from build123d import *

# Parameters (mm, degrees)
SKETCH1_W           = 100
SKETCH1_H           = 1100
BOSS_EXTRUDE1_DEPTH = 200
SKETCH3_W           = 50
SKETCH3_H           = 50
BOSS_EXTRUDE2_DEPTH = 250
FILLET1_R           = 40
BOSS_EXTRUDE3_START = -6
SKETCH4_R           = 20
SKETCH4_R_2         = 15.875
BOSS_EXTRUDE3_DEPTH = 36
CUT_EXTRUDE1_DEPTH  = 20
SKETCH6_W           = 100
SKETCH6_H           = 200
CUT_EXTRUDE2_DEPTH  = 150
SKETCH7_R           = 26
CUT_EXTRUDE3_DEPTH  = 40
SKETCH9_R           = 8
CUT_EXTRUDE5_DEPTH  = 40
SKETCH9_4_R         = 8
CUT_EXTRUDE6_DEPTH  = 40


with BuildPart() as part:
    # Sketch1 → Boss-Extrude1 (new body)
    with BuildSketch(Plane.XY):
        with Locations((-162.86470473, 483.969884115)):
            Rectangle(SKETCH1_W, SKETCH1_H)
    extrude(amount=BOSS_EXTRUDE1_DEPTH)

    # Sketch3 → Boss-Extrude2 (add)
    with BuildSketch(Plane(origin=(-112.86470473, 0, 0), x_dir=(0, 0, -1), z_dir=(1, 0, 0))):
        with Locations((-100, 710.969884115)):
            Rectangle(SKETCH3_W, SKETCH3_H)
    extrude(amount=BOSS_EXTRUDE2_DEPTH)

    # Fillet1
    fillet1_edges = [part.edges().sort_by_distance(p)[0] for p in [
        (-112.86470473, 710.969884115, 75),
        (-112.86470473, 735.969884115, 100),
        (-112.86470473, 710.969884115, 125),
        (-112.86470473, 685.969884115, 100),
    ]]
    fillet(fillet1_edges, radius=FILLET1_R)

    # Sketch4 → Boss-Extrude3 (add)
    # profile 1 of 2: a face of its own
    with BuildSketch(Plane.XY.offset(125).offset(BOSS_EXTRUDE3_START)):
        with BuildLine():
            Line((137.13529527, 722.492751407), (137.13529527, 710.969884115))
            Line((137.13529527, 710.969884115), (137.13529527, 699.447016824))
            Line((137.13529527, 699.447016824), (163.788322175, 699.447016824))
            ThreePointArc((163.788322175, 699.447016824), (160.13529527, 710.969884115), (163.788322175, 722.492751407))
            Line((163.788322175, 722.492751407), (137.13529527, 722.492751407))
        make_face()
    # profile 2 of 2: a face of its own
    with BuildSketch(Plane.XY.offset(125).offset(BOSS_EXTRUDE3_START)):
        with Locations((180.13529527, 710.969884115)):
            Circle(SKETCH4_R)
        with Locations((180.13529527, 710.969884115)):
            Circle(SKETCH4_R_2, mode=Mode.SUBTRACT)
    extrude(amount=-BOSS_EXTRUDE3_DEPTH)

    # Sketch5 → Cut-Extrude1 (cut)
    with BuildSketch(Plane.XZ.offset(66.030115885)):
        with BuildLine():
            ThreePointArc((-162.86470473, 74), (-144.479928419, 81.615223689), (-136.86470473, 100))
            Line((-136.86470473, 100), (-162.86470473, 100))
            Line((-162.86470473, 100), (-162.86470473, 74))
        make_face()
        with BuildLine():
            Line((-162.86470473, 100), (-136.86470473, 100))
            ThreePointArc((-136.86470473, 100), (-144.479928419, 118.384776311), (-162.86470473, 126))
            Line((-162.86470473, 126), (-162.86470473, 100))
        make_face()
        with BuildLine():
            Line((-162.86470473, 74), (-162.86470473, 100))
            Line((-162.86470473, 100), (-188.86470473, 100))
            ThreePointArc((-188.86470473, 100), (-181.24948104, 81.615223689), (-162.86470473, 74))
        make_face()
        with BuildLine():
            Line((-188.86470473, 100), (-162.86470473, 100))
            Line((-162.86470473, 100), (-162.86470473, 126))
            ThreePointArc((-162.86470473, 126), (-181.24948104, 118.384776311), (-188.86470473, 100))
        make_face()
    extrude(amount=-CUT_EXTRUDE1_DEPTH, mode=Mode.SUBTRACT)

    # Sketch6 → Cut-Extrude2 (cut)
    with BuildSketch(Plane.XZ.offset(66.030115885)):
        with Locations((-162.86470473, 100)):
            Rectangle(SKETCH6_W, SKETCH6_H)
    extrude(amount=-CUT_EXTRUDE2_DEPTH, mode=Mode.SUBTRACT)

    # Sketch7 → Cut-Extrude3 (cut)
    with BuildSketch(Plane.XZ.offset(-83.969884115)):
        with Locations(Location((-162.86470473, 100, 0), (0, 0, 270))):
            Circle(SKETCH7_R)
    extrude(amount=-CUT_EXTRUDE3_DEPTH, mode=Mode.SUBTRACT)

    # Sketch9 → Cut-Extrude5 (cut)
    with BuildSketch(Plane(origin=(0, 1033.969884115, 0), x_dir=(1, 0, 0), z_dir=(0, 1, 0))):
        with Locations(Location((-162.86470473, -164.3765, 0), (0, 0, 270))):
            Circle(SKETCH9_R)
    extrude(amount=-CUT_EXTRUDE5_DEPTH, mode=Mode.SUBTRACT)

    # Sketch9_4 → Cut-Extrude6 (cut)
    with BuildSketch(Plane(origin=(0, 1033.969884115, 0), x_dir=(1, 0, 0), z_dir=(0, 1, 0))):
        with Locations(Location((-162.86470473, -35.6235, 0), (0, 0, 270))):
            Circle(SKETCH9_4_R)
    extrude(amount=-CUT_EXTRUDE6_DEPTH, mode=Mode.SUBTRACT)


solid = part.part
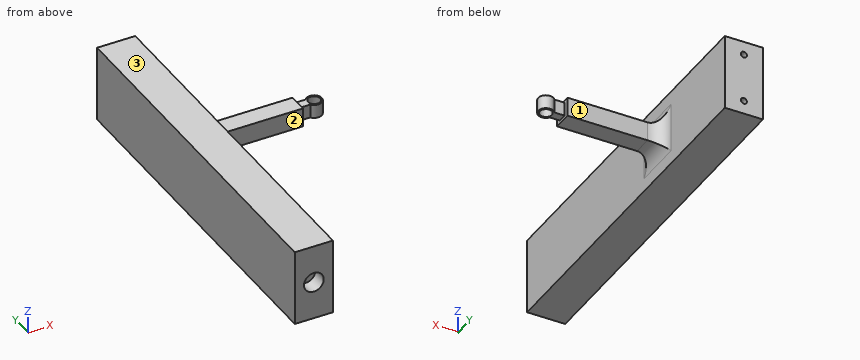
Could you check a few things on this model? Use its own coordinates, in mm. Face numbers are marked on the shaded views. A direction names the side the tool comes from. Give positions to 0.01 mm unless a question says otherwise; leave off trailing zeros. Order: outer loops, then holes, each group sorted by start corner. A loop starts at its lowest first (then second) coordinate and runs counter-clockwise, first axis right, second up. Notation, with made-up numbers: (41, -26.5) - (73, -26.5) arc R9 ccw to (73, -18.5) - close; hole circle Ø8 at (7.5, -39.75). An arc over 180 degrees is marked (long way). One line per item, written item: value. Start each with the question number.
1. Imagine slicing it at C-C on y = 441. List the corners of the cut face in (x, z) for me.
2. For the marked faces 1, 2 and 3, which set-ups out of +Z, -Z, +X, -X, +Y, -Y let a thin tool reach every point of the face, with its end or its side?
3. For P1, Ø8, axis at x = -164.5, z = 167.5, coming from the +Y side; P2, Ø25, axis at x = 43.5, y = 705.5, coming from the -Z side; P3, Ø1, axis at y = 391, z = 56.5, coming from the +X side, each with a flat end and sliding along its axis, tell me the tip position at first contact or that it passes through.
4. Imagine slicing it at B-B on x = 96. List the corners of the cut face in (y, z) for me, plus the area to 3 significant figures.
5. If I drill on probe 1 along X at (y, z) = (625.5, 71); probe 2 along Z at (x, y) = (143, 703); probe 3 along Y at (x, z) = (-162, 86.5), over which ranges is the centre line in solid material (lowest first)?
6. Imagine slicing it at A-A on z = 100. List the corners of the cut face in (x, y) for me (3 decimals).
Values:
1. outline: (-212.86, 0) - (-112.86, 0) - (-112.86, 200) - (-212.86, 200) - close
2. face 1: +Z, -Z, +X, +Y
2. face 2: +Z, -Z, +X, -Y
2. face 3: +Z, +X, -X, +Y, -Y
3. P1: y = 993.97
3. P2: z = 75
3. P3: x = -112.86
4. outline: (685.97, 75) - (735.97, 75) - (735.97, 125) - (685.97, 125) - close
4. area: 2,500 mm²
5. probe 1: -212.86 to -112.86
5. probe 2: 83 to 119
5. probe 3: 123.97 to 1033.97
6. outline: (-212.865, 83.97) - (-188.865, 83.97) - (-188.865, 123.97) - (-136.865, 123.97) - (-136.865, 83.97) - (-112.865, 83.97) - (-112.865, 645.97) arc R40 cw to (-72.865, 685.97) - (137.135, 685.97) - (137.135, 699.447) - (163.788, 699.447) arc R20 ccw (long way) to (163.788, 722.493) - (137.135, 722.493) - (137.135, 735.97) - (-72.865, 735.97) arc R40 cw to (-112.865, 775.97) - (-112.865, 1033.97) - (-212.865, 1033.97) - close; hole circle Ø31.75 at (180.135, 710.97)
